from build123d import *

# Parameters (mm, degrees)
F0_W     = 133.8296830654
F0_H     = 30.2196051925
F0_R     = 12.6806101672
F0_R_2   = 13.1338475118
F0_R_3   = 13.2147961645
F1_DEPTH = 25.4
F2_R     = 9.5291524703
F2_R_2   = 10.876810803
F2_R_3   = 10.4970200843
F2_R_4   = 10.5638834355
F3_DEPTH = 30.48


with BuildPart() as f1:
    # F0 (on Top) → F1 (new body)
    with BuildSketch(Plane.XY):
        Rectangle(F0_W, F0_H)
        with Locations((-49.6464930475, 0)):
            Circle(F0_R, mode=Mode.SUBTRACT)
        Circle(F0_R_2, mode=Mode.SUBTRACT)
        with Locations((45.0416021049, 0)):
            Circle(F0_R_3, mode=Mode.SUBTRACT)
        with Locations((45.0416021049, 0)):
            Circle(F0_R_3)
        Circle(F0_R_2)
        with Locations((-49.6464930475, 0)):
            Circle(F0_R)
    extrude(amount=F1_DEPTH)

    # F2 (on face) → F3 (join)
    with BuildSketch(Plane(origin=(0, 0, 0), x_dir=(1, 0, 0), z_dir=(0, 0, -1))):
        with Locations((-56.8416379392, 0)):
            Circle(F2_R)
        with Locations((-25.7586147636, 0)):
            Circle(F2_R_2)
        with Locations((20.290305838, 0)):
            Circle(F2_R_3)
        with Locations((54.25138399, 0)):
            Circle(F2_R_4)
    extrude(amount=-F3_DEPTH)


solid = f1.part
Design review of the part built by this model. Coordinates are the model's own, in mm. A direction names the side the tool comes from. Round coordinates to 2 decimals unless told otherwise and drop trailing zeros. Loops run counter-clockwise (first coordinate to the right, second up) from the corner with the lowest first, then second, coordinate; pieces in that order, holes last. Notation, with made-up numbers: (-4, -24) - (2, -24) arc R13 cw to (2, -7) - close; hole circle Ø5 at (67.25, 37.25). An arc over 180 degrees is marked (long way). One line per item, written item: value. Start each with the question number.
1) Consider section D-D on y = 7.5. Give the boundary of the cut face in (x, z), then the cut area to 3 significant figures.
2) To check wall thickness, follow L1, parallel to Z at x = -51, y = 10; L2, parallel to Y at x = -60, z = 29.5; L3, parallel to Y at x = 26, z = 27.5. State the ranges of each line that lie inside material, in increasing order. Write a range as from..to.
3) For faces 5 (the flat face through (-1, 15.11, 13)), 6 (the cylindrical face through (-15.384, -3.267, 27.904)), list the 3-axis set-ups (+Z, -Z, +X, -X, +Y, -Y) from which the entire face can be reached by the end or side of a thin tool; tool diameter is ignored.
4) Draft analysis for pull direction X (two halves, no side actions). For faces 1 (the flat face through (-66.915, 0, 13)), 2 (the flat face through (66.915, 0, 13)), 3 (the flat face through (-26, 0, 30.48)), 4 (the cylindrical face through (-66.36, -0.42, 27.9)), state which applies: +X half, -X half, draft (parallel to the pull), parting line (faces both ways), or undercut.
5) Consider section C-C on x = 7.5. Give the boundary of the cut face in (y, z), then the cut area to 3 significant figures.
6) Consider section B-B on y = 0. Give the boundary of the cut face in (x, z).
7) Consider section A-A on z = 27. Give the boundary of the cut face in (x, y), then the cut area to 3 significant figures.
8) Insertion check: pin 1 Ø1.5 at (x, y) = (29, 1) entering from -Z; pin 2 Ø2 at (y, z) = (-5, 27) entering from +X; pin 3 Ø1 at (x, y) = (8.5, 5.5) entering from +Z. Each pin has a flat end and moves straight along its axis. Give the tip position at first contact, or say it passes through.
Reported:
1. outline: (-66.91, 0) - (66.91, 0) - (66.91, 25.4) - (61.69, 25.4) - (61.69, 30.48) - (46.81, 30.48) - (46.81, 25.4) - (27.63, 25.4) - (27.63, 30.48) - (12.95, 30.48) - (12.95, 25.4) - (-17.88, 25.4) - (-17.88, 30.48) - (-33.64, 30.48) - (-33.64, 25.4) - (-50.96, 25.4) - (-50.96, 30.48) - (-62.72, 30.48) - (-62.72, 25.4) - (-66.91, 25.4) - close
1. area: 3,690 mm^2
2. L1: z = 0..25.4
2. L2: y = -8.99..8.99
2. L3: y = -8.81..8.81
3. face 5: +Z, -Z, +X, -X, +Y
3. face 6: +Z
4. face 1: -X half
4. face 2: +X half
4. face 3: draft
4. face 4: undercut
5. outline: (-15.11, 0) - (15.11, 0) - (15.11, 25.4) - (-15.11, 25.4) - close
5. area: 768 mm^2
6. outline: (-66.91, 0) - (66.91, 0) - (66.91, 25.4) - (64.82, 25.4) - (64.82, 30.48) - (43.69, 30.48) - (43.69, 25.4) - (30.79, 25.4) - (30.79, 30.48) - (9.79, 30.48) - (9.79, 25.4) - (-14.88, 25.4) - (-14.88, 30.48) - (-36.64, 30.48) - (-36.64, 25.4) - (-47.31, 25.4) - (-47.31, 30.48) - (-66.37, 30.48) - (-66.37, 25.4) - (-66.91, 25.4) - close
7. outline: circle Ø19.06 at (-56.84, 0); circle Ø21.75 at (-25.76, 0); circle Ø20.99 at (20.29, 0); circle Ø21.13 at (54.25, 0)
7. area: 1,350 mm^2
8. pin 1: stops at z = 0
8. pin 2: stops at x = 64.03
8. pin 3: stops at z = 25.4
